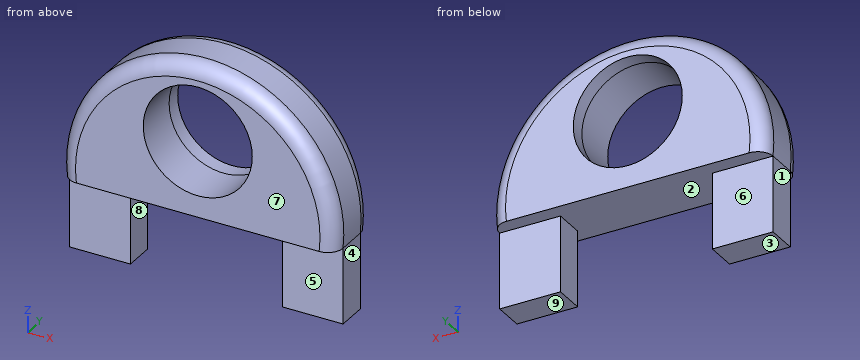
from build123d import *
from build123d import SkipClean  # not in build123d's __all__

# Parameters (mm, degrees)
F0_R        = 3.59
F1_DEPTH    = 2
F2_R        = 3.59
F3_DEPTH    = 1
F4_R        = 3.59
F5_DEPTH    = 1
F7_T3_ANGLE = 223.7642380541
F7_T6_ANGLE = 223.7642380541


# Not quite as in the source:
# - a fillet or chamfer that OpenCascade refuses, or shapes differently, is made with other operations: its cross-section is extruded or revolved along the edge and cut away or added
# - a feature of the source that left no trace in its solid (it failed there, or was rolled back) is left out


with BuildPart() as f1:
    # F0 (on Front) → F1 (new body)
    with BuildSketch(Plane.XZ):
        with BuildLine():
            Line((-28.8239947557, 12.7150369808), (-28.8239947557, 17.7150369808))
            Line((-28.8239947557, 17.7150369808), (-18.8239947557, 17.7150369808))
            Line((-18.8239947557, 17.7150369808), (-18.8239947557, 12.7150369808))
            Line((-18.8239947557, 12.7150369808), (-14.8239947557, 12.7150369808))
            Line((-14.8239947557, 12.7150369808), (-14.8239947557, 17.7150369808))
            ThreePointArc((-14.8239947557, 17.7150369808), (-23.8239947557, 27.7150369808), (-32.8239947557, 17.7150369808))
            Line((-32.8239947557, 17.7150369808), (-32.8239947557, 12.7150369808))
            Line((-32.8239947557, 12.7150369808), (-28.8239947557, 12.7150369808))
        make_face()
        with Locations((-23.8239947557, 22.7150369808)):
            Circle(F0_R, mode=Mode.SUBTRACT)
    extrude(amount=F1_DEPTH)

    # F2 (on face) → F3 (join)
    with BuildSketch(Plane.XZ.offset(2)):
        with BuildLine():
            Line((-32.8239947557, 17.7150369808), (-28.8239947557, 17.7150369808))
            Line((-28.8239947557, 17.7150369808), (-18.8239947557, 17.7150369808))
            Line((-18.8239947557, 17.7150369808), (-14.8239947557, 17.7150369808))
            ThreePointArc((-14.8239947557, 17.7150369808), (-23.8239947557, 27.7150369808), (-32.8239947557, 17.7150369808))
        make_face()
        with Locations((-23.8239947557, 22.7150369808)):
            Circle(F2_R, mode=Mode.SUBTRACT)
    extrude(amount=F3_DEPTH)

    # F4 (on face) → F5 (join)
    with BuildSketch(Plane(origin=(0, 0, 0), x_dir=(-1, 0, 0), z_dir=(0, 1, 0))):
        with BuildLine():
            Line((14.8239947557, 17.7150369808), (18.8239947557, 17.7150369808))
            Line((18.8239947557, 17.7150369808), (28.8239947557, 17.7150369808))
            Line((28.8239947557, 17.7150369808), (32.8239947557, 17.7150369808))
            ThreePointArc((32.8239947557, 17.7150369808), (23.8239947557, 27.7150369808), (14.8239947557, 17.7150369808))
        make_face()
        with Locations((23.8239947557, 22.7150369808)):
            Circle(F4_R, mode=Mode.SUBTRACT)
    with SkipClean():  # cleaning this boolean's faces spoils the solid; the shape is the same uncleaned
        extrude(amount=F5_DEPTH)

    # F7: fillet of radius 1 on 2 edges, made by hand


with BuildPart() as f7_tool1:
    # F7_s2 → F7_t3 (revolve)
    with BuildSketch(Plane(origin=(3.1459864442, 0, 7.8329498468), x_dir=(0, 1, 0), z_dir=(-0.3726982036, 0, -0.9279526114))):
        with BuildLine():
            ThreePointArc((-2, -20.0139639005), (-2.7071067812, -20.3068571193), (-3, -21.0139639005))
            Line((-3, -21.0139639005), (-3, -20.0139639005))
            Line((-3, -20.0139639005), (-2, -20.0139639005))
        make_face()
    revolve(axis=Axis((-23.8239947557, -3, 18.6650369808), (0, -1, 0)), revolution_arc=F7_T3_ANGLE)


with BuildPart() as f7_tool4:
    # F7_s5 → F7_t6 (revolve)
    with BuildSketch(Plane(origin=(-9.7644804416, 0, 24.3118293528), x_dir=(0, 1, 0), z_dir=(0.3726982036, 0, -0.9279526114))):
        with BuildLine():
            ThreePointArc((0, -24.2011123962), (0.7071067812, -23.9082191774), (1, -23.2011123962))
            Line((1, -23.2011123962), (1, -24.2011123962))
            Line((1, -24.2011123962), (0, -24.2011123962))
        make_face()
    revolve(axis=Axis((-23.8239947557, 1, 18.6650369808), (0, 1, 0)), revolution_arc=F7_T6_ANGLE)


with BuildPart() as f1_1:
    add(f1.part, clean=False)

    # F7_t7: cut F7_tool1, F7_tool4
    add([f7_tool1.part, f7_tool4.part], mode=Mode.SUBTRACT)


solid = f1_1.part
Input: part model. Units: mm. Frame: model coordinates. Face numbers are marked on the shaded views. A direction names the side the tool comes from. Give positions to 0.01 mm unless a question says otherwise; leave off trailing zeros. Write each loop counter-clockwise with the first axis right and the second up, starting at its lowest first coordinate (ties: lowest second). Pieces come first, ordered by that corner, then holes. Notation, with made-up numbers: (75, 41.25) -> (107, 41.25) arc R9 cw to (107, 54.25) -> close; hole circle Ø8 at (36, 51.25). An arc over 180 degrees is marked (long way). Use one line per item in the form item = value. Start each with the question number.
1) Draft query along X for the marked faces 1, 2, 3 and 4. Return one class per face: pulls with the +X half, pulls with the -X half, needs draft (parallel to the pull), parting line crosses it, or undercut.
2) Ray query, probe 1 along X at (y, z) = (-0.85, 15.75); probe 2 along Y at (x, z) = (-31.5, 16.5); probe 3 along X at (y, z) = (-2.4, 24.5). Return the intervals inside material, ascending. Write a range as from..to.
3) Pin query (flat end, axial travel): pin 1 (1.6 mm diameter, centred on y = -1, z = 15.5, fed in from +X); pin 2 (1.2 mm diameter, centred on x = -16, z = 14.5, fed in from -Y); pin 3 (2 mm diameter, centred on x = -27, y = -1.5, fed in from -Z); pin 4 (5.5 mm diameter, centred on x = -23.82, z = 22.72, fed in from -Y). Return the tip coordinate at first contact, or that it passes through.
4) Section query A-A on z = 15.5. Return the cut outline in (x, y), then the cut area to 3 significant figures.
5) Section query B-B on y = -1.75. Return the cut outline in (x, z).
6) Section query D-D on y = -2.8. Return the cut outline in (x, z).
7) Set-up query: the marked faces 5, 6, 7, 8 and 9. Return all of +Z, -Z, +X, -X, +Y, -Y with unobstructed straight access to the full face (end or side cutting, diameter ignored); none if empty.
Outcome:
q1.face_1 = pulls with the -X half
q1.face_2 = undercut
q1.face_3 = needs draft
q1.face_4 = pulls with the +X half
q2.probe_1 = -32.82..-28.82, -18.82..-14.82
q2.probe_2 = -2..0
q2.probe_3 = -30.63..-26.94, -20.71..-17.02
q3.pin_1 = -14.82
q3.pin_2 = -2
q3.pin_3 = 17.72
q3.pin_4 = through
q4.outline = (-32.82, -2) -> (-28.82, -2) -> (-28.82, 0) -> (-32.82, 0) -> close; (-18.82, -2) -> (-14.82, -2) -> (-14.82, 0) -> (-18.82, 0) -> close
q4.area = 16.0 mm^2
q5.outline = (-32.82, 12.72) -> (-28.82, 12.72) -> (-28.82, 17.72) -> (-18.82, 17.72) -> (-18.82, 12.72) -> (-14.82, 12.72) -> (-14.82, 17.72) arc R9.05 ccw (long way) to (-32.82, 17.72) -> close; hole circle Ø7.18 at (-23.82, 22.72)
q6.outline = (-32.42, 17.72) -> (-15.23, 17.72) arc R8.65 ccw (long way) to start; hole circle Ø7.18 at (-23.82, 22.72)
q7.face_5 = -Z, +X, -X, -Y
q7.face_6 = -Z, +X, -X, +Y
q7.face_7 = +Z, -Z, +X, -X, -Y
q7.face_8 = -Z, +Y, -Y
q7.face_9 = -Z, +X, -X, +Y, -Y
